Geometry check sheet. Reference: the model listing, model coordinates, mm. Face numbers are marked on the shaded views. A direction names the side the tool comes from. Coordinates: 2 decimals unless noted, no trailing zeros. Order: outer loops, then holes, each group sorted by start corner. A loop starts at its lowest first (then second) coordinate and runs counter-clockwise, first axis right, second up. Notation, with made-up numbers: M -39.75,-13 L -18.75,-13 A23 ccw -18.75,21 Z; hole C 4,58.5 d5. An arc over 180 degrees is marked long. Use CSV: the item, a comma, the result in double quotes. Start each with the question number.
```python
from build123d import *

# Parameters (mm, degrees)
F1_DEPTH = 8
F2_W     = 6.5
F2_H     = 6.5
F3_DEPTH = 1.3
F4_R     = 3.1
F5_DEPTH = 6.3


with BuildPart() as f1:
    # F0 (on Top) → F1 (new body)
    with BuildSketch(Plane.XY):
        Polygon((-0.430666, 6.157663), (-11.430666, 6.157663), (-11.430666, -19.592337), (8.569334, -19.592337), (8.569334, 6.157663), (8.569334, 9.007663), (-0.430666, 9.007663), align=None)
    extrude(amount=F1_DEPTH)

    # F2 (on face) → F3 (join)
    with BuildSketch(Plane(origin=(0, 9.007663, 0), x_dir=(-1, 0, 0), z_dir=(0, 1, 0))):
        with Locations((-3.819334, 4.75)):
            Rectangle(F2_W, F2_H)
    extrude(amount=F3_DEPTH)

    # F4 (on face) → F5 (join)
    with BuildSketch(Plane(origin=(0, 10.307663, 0), x_dir=(-1, 0, 0), z_dir=(0, 1, 0))):
        with Locations((-3.819334, 4.75)):
            Circle(F4_R)
    extrude(amount=F5_DEPTH)


solid = f1.part
```
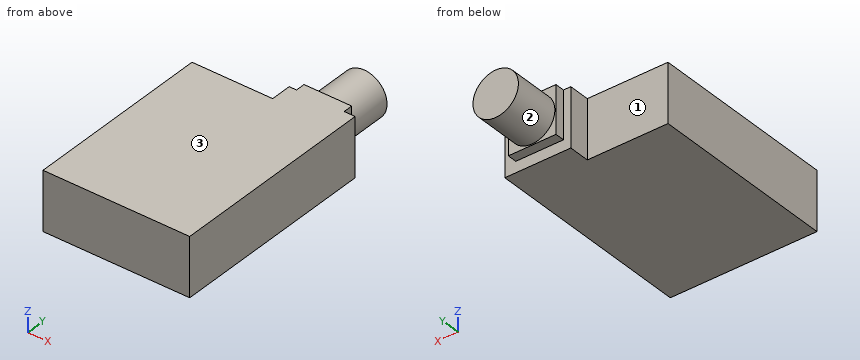
1) Section check A-A on z = 4.75. Record the boundary of the cut face in (x, y), then the cut area to 3 significant figures.
2) Section check C-C on x = -7.5. Record the boundary of the cut face in (y, z).
3) Section check B-B on x = 2.5. Record the boundary of the cut face in (y, z).
4) Set-up check for the marked faces 1, 2 and 3: record each of +Z, -Z, +X, -X, +Y, -Y from which the full face is reachable in a straight line by a thin tool's end or side.
5) Gauge pin test, flat end, axial feed: P1, Ø2, axis at y = 11, z = 4, coming from the -X side. Record the tip position at first contact, or that the pin passes through.
6) Material ranges on line 1 along Z through (x, y) = (3.75, 14); line 2 along Y through (x, z) = (-3, 4); line 3 along X through (y, z) = (6.5, 1), recorded low to high.
Results are:
1,outline,"M -11.43,-19.59 L 8.57,-19.59 L 8.57,9.01 L 7.07,9.01 L 7.07,10.31 L 6.92,10.31 L 6.92,16.61 L 0.72,16.61 L 0.72,10.31 L 0.57,10.31 L 0.57,9.01 L -0.43,9.01 L -0.43,6.16 L -11.43,6.16 Z"
1,area,"588 mm²"
2,outline,"M -19.59,0 L 6.16,0 L 6.16,8 L -19.59,8 Z"
3,outline,"M -19.59,0 L 9.01,0 L 9.01,1.5 L 10.31,1.5 L 10.31,1.94 L 16.61,1.94 L 16.61,7.56 L 10.31,7.56 L 10.31,8 L -19.59,8 Z"
4,face 1,"+Z, -Z, -X, +Y"
4,face 2,"+Y"
4,face 3,"+Z, +X, -X, +Y, -Y"
5,P1,"stops at x = 0.57"
6,line 1,"z = 1.65 to 7.85"
6,line 2,"y = -19.59 to 6.16"
6,line 3,"x = -0.43 to 8.57"
